```python
from build123d import *

# Parameters (mm, degrees)
CROQUIS1_W              = 63.5
CROQUIS1_H              = 63.5
CROQUIS1_W_2            = 59.7
CROQUIS1_H_2            = 59.7
SALIENTE_EXTRUIR1_DEPTH = 140
CROQUIS2_W              = 59.7
CROQUIS2_H              = 59.7
SALIENTE_EXTRUIR2_DEPTH = 1.9
CROQUIS3_W              = 59.7
CROQUIS3_H              = 59.7
SALIENTE_EXTRUIR3_DEPTH = 1.9


with BuildPart() as part:
    # Croquis1 → Saliente-Extruir1 (new body)
    with BuildSketch(Plane.XY):
        with Locations((31.75, -31.75)):
            Rectangle(CROQUIS1_W, CROQUIS1_H)
        with Locations((31.75, -31.75)):
            Rectangle(CROQUIS1_W_2, CROQUIS1_H_2, mode=Mode.SUBTRACT)
    extrude(amount=SALIENTE_EXTRUIR1_DEPTH)

    # Croquis2 → Saliente-Extruir2 (add)
    with BuildSketch(Plane.XY.offset(140)):
        with Locations((31.75, -31.75)):
            Rectangle(CROQUIS2_W, CROQUIS2_H)
    extrude(amount=-SALIENTE_EXTRUIR2_DEPTH)

    # Croquis3 → Saliente-Extruir3 (add)
    with BuildSketch(Plane(origin=(0, 0, 0), x_dir=(-1, 0, 0), z_dir=(0, 0, -1))):
        with Locations((-31.75, -31.75)):
            Rectangle(CROQUIS3_W, CROQUIS3_H)
    extrude(amount=-SALIENTE_EXTRUIR3_DEPTH)


solid = part.part
```
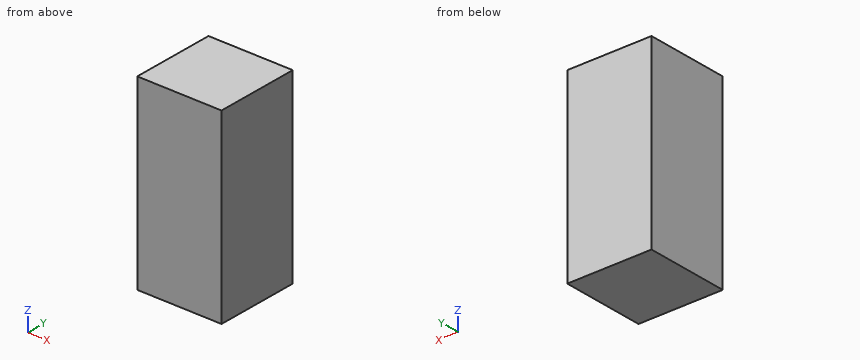
Build history of the part. All positions in model axes, mm. Give positions to 0.01 mm unless a question says otherwise; leave off trailing zeros. Loops run counter-clockwise (first coordinate to the right, second up) from the corner with the lowest first, then second, coordinate; pieces in that order, holes last. Notation, with made-up numbers: (38, -9) -> (62, -9) arc R15 cw to (62, -5) -> close; hole circle Ø6 at (-34.5, 11). An arc over 180 degrees is marked (long way). One line per question, with ' | ' between items. Start each with the question number.
1) Cut at A-A (z = 64). Give the cut face in (x, y), plus the area to 3 significant figures.
2) Cut at B-B (y = -13.5). Give the cut face in (x, z), plus the area to 3 significant figures.
3) Probe L1, parallel to X at y = -16.5, z = 10; L2, parallel to Y at x = 37, z = 50; L3, parallel to Z at x = 22, y = -27. List the from-to ranges inside material, lowest first.
4) Pin check, flat tip, straight feed: pin 1 (18 mm diameter, centred on y = -33, z = 84.5, fed in from -X). Stop position of the tip, or through.
Return value:
1) outline: (0, -63.5) -> (63.5, -63.5) -> (63.5, 0) -> (0, 0) -> close; hole (1.9, -61.6) -> (61.6, -61.6) -> (61.6, -1.9) -> (1.9, -1.9) -> close | area: 468 mm^2
2) outline: (0, 0) -> (63.5, 0) -> (63.5, 140) -> (0, 140) -> close; hole (1.9, 1.9) -> (61.6, 1.9) -> (61.6, 138.1) -> (1.9, 138.1) -> close | area: 759 mm^2
3) L1: 0 to 1.9, 61.6 to 63.5 | L2: -63.5 to -61.6, -1.9 to 0 | L3: 0 to 1.9, 138.1 to 140
4) pin 1: x = 0
